Job drawing, mm, ordinate dimensions from the low corner. One solid piece. Give positions to 0.01 mm unless a question says otherwise; leave off trailing zeros. Write each loop counter-clockwise with the first axis right and the second up, starting at its lowest first coordinate (ties: lowest second). Pieces come first, ordered by that corner, then holes. Notation, with made-up numbers: (-1, 7.25) - (50, 7.25) arc R13 ccw to (50, 32.25) - close; hole circle Ø1 at (-33, 55). An arc over 180 degrees is marked (long way). Answer in a Markdown table with one row per item. Add a question column.
1. Band-saw the part on A-A on y = 23. Write the cut outline in (x, z), plus the area to 4 significant figures.
2. Drop flat-ended pins along their axis: pin 1 Ø4 at (y, z) = (32.5, 16) entering from +X; pin 2 Ø4 at (y, z) = (57, 16) entering from +X; pin 3 Ø12 at (y, z) = (84, 20.5) entering from +X. Give the stop position or say it passes through.
3. Band-saw the part on B-B on x = 101.5. Write the cut outline in (y, z).
4. Band-saw the part on C-C on z = 12.25. State how many separate pieces and enclosed holes the cut face has, plus the area to 3 significant figures.
5. Probe line 1 along X through (y, z) = (32, 3); line 2 along Y through (x, z) = (58.5, 21.25) (1 decimal); line 3 along Y through (x, z) = (41, 24.25). List the from-to ranges inside material, lowest first.
6. Pull direction X, two halves, no side cores. Call the marked faces 1, 2, 3 and 4: released by +X, released by -X, zero draft, split by the parting line, or undercut.
7. Band-saw the part on D-D on y = 75. Write the cut outline in (x, z).
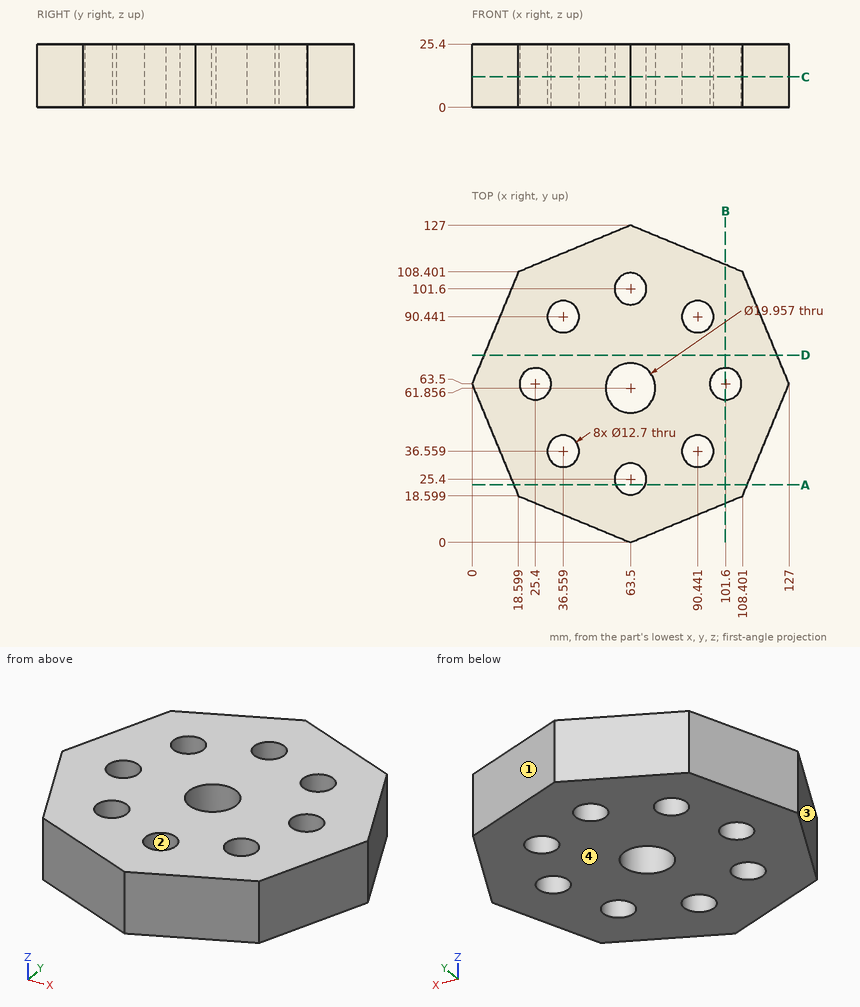
Values:
| question | item | result |
|---|---|---|
| 1 | outline | (16.78, 0) - (57.62, 0) - (57.62, 25.4) - (16.78, 25.4) - close; (69.38, 0) - (110.22, 0) - (110.22, 25.4) - (69.38, 25.4) - close |
| 1 | area | 2,075 mm² |
| 2 | pin 1 | stops at x = 114.99 |
| 2 | pin 2 | stops at x = 125.14 |
| 2 | pin 3 | stops at x = 120.99 |
| 3 | outline | (15.74, 0) - (57.15, 0) - (57.15, 25.4) - (15.74, 25.4) - close; (69.85, 0) - (111.26, 0) - (111.26, 25.4) - (69.85, 25.4) - close |
| 4 | separate pieces | 1 |
| 4 | enclosed holes | 9 |
| 4 | area | 10,100 mm² |
| 5 | line 1 | x = 13.05 to 32.14, 40.98 to 86.02, 94.86 to 113.95 |
| 5 | line 2 | y = 2.1 to 21.5, 29.3 to 53.2, 70.5 to 97.7, 105.5 to 124.9 |
| 5 | line 3 | y = 9.32 to 32.02, 41.1 to 85.9, 94.98 to 117.68 |
| 6 | face 1 | released by +X |
| 6 | face 2 | undercut |
| 6 | face 3 | released by -X |
| 6 | face 4 | zero draft |
| 7 | outline | (4.76, 0) - (122.24, 0) - (122.24, 25.4) - (4.76, 25.4) - close |
